Input: part model. Units: mm. Frame: model coordinates. Face numbers are marked on the shaded views. Give positions to 0.01 mm unless a question says otherwise; leave off trailing zeros. Write each loop counter-clockwise with the first axis right and the second up, starting at its lowest first coordinate (ties: lowest second). Pieces come first, ordered by that corner, then holes. Notation, with made-up numbers: (4.25, -30.5) - (41.25, -30.5) arc R15 ccw to (41.25, -11.5) - close; hole circle Ø2 at (30.25, 75). An arc over 180 degrees is marked (long way). Use a Markdown table: item, result. Add a question column.
1. Mould query, pull axis X, two halves, no side actions, for the marked faces 1 and 2. Classes: released by +X, released by -X, zero draft, split by the parting line, or undercut.
2. Pin query (flat end, axial travel): pin 1 (2 mm diameter, centred on x = 7.5, z = -20, fed in from +Y); pin 2 (0.5 mm diameter, centred on y = 1, z = -43, fed in from +X); pin 3 (1.7 mm diameter, centred on x = 1, y = 1, fed in from -Z). Return the tip coordinate at first contact, or that it passes through.
3. Section query C-C, the plane y = 3.75. Return loops of the section in (x, z), plus the area to 3 significant figures.
4. Material intervals for probe 1 along X at (y, z) = (2, -20.5); probe 2 along X at (y, z) = (0.7, 0) (1 decimal); probe 3 along Y at (x, z) = (-17, -18), sorted ascending.
5. Section query A-A, the plane z = 0. Count the separate pieces of the cut face and the enclosed holes in it, plus the area to 3 significant figures.
6. Section query B-B, the plane x = 0. Return loops of the section in (y, z) (1 decimal), plus the area to 3 significant figures.
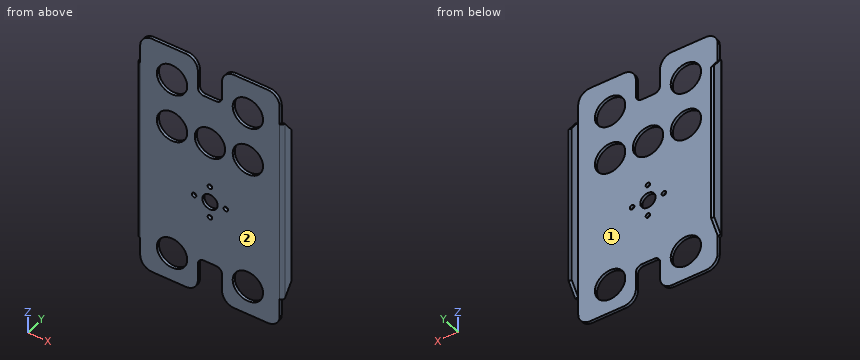
```python
from build123d import *

# Parameters (mm, degrees)
SKETCH1_R               = 7.9375
SKETCH1_R_2             = 4.0005
SKETCH1_R_3             = 1.1938
EXTRUDE1_DEPTH          = 1.524
EXTRUDE2_DEPTH          = 6.35
CUT_EXTRUDE1_DEPTH      = 39.1
CUT_EXTRUDE1_DEPTH_BACK = 39.1
FILLET1_R               = 1.5875


with BuildPart() as part:
    # Sketch1 → Extrude1 (new body)
    with BuildSketch(Plane(origin=(0, 0, 0), x_dir=(1, 0, 0), z_dir=(0, 1, 0))):
        with BuildLine():
            Line((36.4998, -62.3062), (36.4998, 36.1188))
            Line((36.4998, 36.1188), (36.4998, 39.2938))
            Line((36.4998, 39.2938), (36.4998, 45.6438))
            ThreePointArc((36.4998, 45.6438), (34.639928061, 50.133928061), (30.1498, 51.9938))
            Line((30.1498, 51.9938), (23.7998, 51.9938))
            Line((23.7998, 51.9938), (12.7, 51.9938))
            ThreePointArc((12.7, 51.9938), (8.209871939, 50.133928061), (6.35, 45.6438))
            Line((6.35, 45.6438), (6.35, 36.5252))
            ThreePointArc((6.35, 36.5252), (5.42006403, 34.28013597), (3.175, 33.3502))
            Line((3.175, 33.3502), (-3.175, 33.3502))
            ThreePointArc((-3.175, 33.3502), (-5.42006403, 34.28013597), (-6.35, 36.5252))
            Line((-6.35, 36.5252), (-6.35, 45.6438))
            ThreePointArc((-6.35, 45.6438), (-8.209871939, 50.133928061), (-12.7, 51.9938))
            Line((-12.7, 51.9938), (-23.7998, 51.9938))
            Line((-23.7998, 51.9938), (-30.1498, 51.9938))
            ThreePointArc((-30.1498, 51.9938), (-34.639928061, 50.133928061), (-36.4998, 45.6438))
            Line((-36.4998, 45.6438), (-36.4998, 39.2938))
            Line((-36.4998, 39.2938), (-36.4998, 36.1188))
            Line((-36.4998, 36.1188), (-36.4998, -62.3062))
            Line((-36.4998, -62.3062), (-36.4998, -68.6562))
            ThreePointArc((-36.4998, -68.6562), (-34.639928061, -73.146328061), (-30.1498, -75.0062))
            Line((-30.1498, -75.0062), (-23.7998, -75.0062))
            Line((-23.7998, -75.0062), (-12.7, -75.0062))
            ThreePointArc((-12.7, -75.0062), (-8.209871939, -73.146328061), (-6.35, -68.6562))
            Line((-6.35, -68.6562), (-6.35, -59.5376))
            ThreePointArc((-6.35, -59.5376), (-5.42006403, -57.29253597), (-3.175, -56.3626))
            Line((-3.175, -56.3626), (3.175, -56.3626))
            ThreePointArc((3.175, -56.3626), (5.42006403, -57.29253597), (6.35, -59.5376))
            Line((6.35, -59.5376), (6.35, -68.6562))
            ThreePointArc((6.35, -68.6562), (8.209871939, -73.146328061), (12.7, -75.0062))
            Line((12.7, -75.0062), (23.7998, -75.0062))
            Line((23.7998, -75.0062), (30.1498, -75.0062))
            ThreePointArc((30.1498, -75.0062), (34.639928061, -73.146328061), (36.4998, -68.6562))
            Line((36.4998, -68.6562), (36.4998, -62.3062))
        make_face()
        with Locations(Location((19.8374, -57.531, 0), (0, 0, 270))):  # turned: the seam where the file's is
            Circle(SKETCH1_R, mode=Mode.SUBTRACT)
        with Locations(Location((19.8374, -32.131, 0), (0, 0, 270))):  # turned: the seam where the file's is
            Circle(SKETCH1_R, mode=Mode.SUBTRACT)
        with Locations(Location((0, 0, 0), (0, 0, 270))):  # turned: the seam where the file's is
            Circle(SKETCH1_R_2, mode=Mode.SUBTRACT)
        with Locations(Location((8.3312, 0, 0), (0, 0, 270))):  # turned: the seam where the file's is
            Circle(SKETCH1_R_3, mode=Mode.SUBTRACT)
        with Locations(Location((0, -8.3312, 0), (0, 0, 270))):  # turned: the seam where the file's is
            Circle(SKETCH1_R_3, mode=Mode.SUBTRACT)
        with Locations(Location((0, 8.3312, 0), (0, 0, 270))):  # turned: the seam where the file's is
            Circle(SKETCH1_R_3, mode=Mode.SUBTRACT)
        with Locations(Location((-8.3312, 0, 0), (0, 0, 270))):  # turned: the seam where the file's is
            Circle(SKETCH1_R_3, mode=Mode.SUBTRACT)
        with Locations(Location((19.8374, 36.9062, 0), (0, 0, 270))):  # turned: the seam where the file's is
            Circle(SKETCH1_R, mode=Mode.SUBTRACT)
        with Locations(Location((0, -32.131, 0), (0, 0, 270))):  # turned: the seam where the file's is
            Circle(SKETCH1_R, mode=Mode.SUBTRACT)
        with Locations(Location((-19.8374, 36.9062, 0), (0, 0, 270))):  # turned: the seam where the file's is
            Circle(SKETCH1_R, mode=Mode.SUBTRACT)
        with Locations(Location((-19.8374, -32.131, 0), (0, 0, 270))):  # turned: the seam where the file's is
            Circle(SKETCH1_R, mode=Mode.SUBTRACT)
        with Locations(Location((-19.8374, -57.531, 0), (0, 0, 270))):  # turned: the seam where the file's is
            Circle(SKETCH1_R, mode=Mode.SUBTRACT)
    extrude(amount=EXTRUDE1_DEPTH)

    # Sketch1_3 → Extrude2 (add)
    with BuildSketch(Plane(origin=(0, 0, 0), x_dir=(1, 0, 0), z_dir=(0, 1, 0))):
        Polygon((36.4998, 36.1188), (36.4998, -59.1312), (38.1, -59.1312), (38.1, 29.7688), (38.1, 36.1188), align=None)
        Polygon((-38.1, -59.1312), (-36.4998, -59.1312), (-36.4998, 36.1188), (-38.1, 36.1188), (-38.1, 29.7688), align=None)
    extrude(amount=EXTRUDE2_DEPTH)

    # Sketch2 → Cut-Extrude1 (cut, two sides)
    with BuildSketch(Plane(origin=(0, 0, 0), x_dir=(0, 0, -1), z_dir=(1, 0, 0))) as cut_extrude1_sk:
        Polygon((-59.1312, 6.35), (-59.1312, 1.524), (-52.7812, 6.35), align=None)
        Polygon((36.1188, 6.35), (29.7688, 6.35), (36.1188, 1.524), align=None)
    extrude(amount=CUT_EXTRUDE1_DEPTH, mode=Mode.SUBTRACT)
    extrude(cut_extrude1_sk.sketch, amount=-CUT_EXTRUDE1_DEPTH_BACK, mode=Mode.SUBTRACT)

    # Fillet1
    fillet1_edges = [part.edges().sort_by_distance(p)[0] for p in [
        (38.1, 0, 11.5062),
        (-38.1, 0, 11.5062),
    ]]
    fillet(fillet1_edges, radius=FILLET1_R)


solid = part.part
```
Result sheet:
| question | item | result |
|---|---|---|
| 1 | face 1 | undercut |
| 1 | face 2 | zero draft |
| 2 | pin 1 | stops at y = 1.52 |
| 2 | pin 2 | stops at x = 36.5 |
| 2 | pin 3 | stops at z = -33.35 |
| 3 | outline | (-38.1, -33.19) - (-36.5, -33.19) - (-36.5, 56.2) - (-38.1, 56.2) - close; (36.5, -33.19) - (38.1, -33.19) - (38.1, 56.2) - (36.5, 56.2) - close |
| 3 | area | 286 mm² |
| 4 | probe 1 | x = -38.1 to -36.5, 36.5 to 38.1 |
| 4 | probe 2 | x = -37.8 to -9.5, -7.1 to -4, 4 to 7.1, 9.5 to 37.8 |
| 4 | probe 3 | y = 0 to 1.52 |
| 5 | separate pieces | 4 |
| 5 | enclosed holes | 0 |
| 5 | area | 111 mm² |
| 6 | outline | (0, -33.4) - (1.5, -33.4) - (1.5, -9.5) - (0, -9.5) - close; (0, -7.1) - (1.5, -7.1) - (1.5, -4) - (0, -4) - close; (0, 4) - (1.5, 4) - (1.5, 7.1) - (0, 7.1) - close; (0, 9.5) - (1.5, 9.5) - (1.5, 24.2) - (0, 24.2) - close; (0, 40.1) - (1.5, 40.1) - (1.5, 56.4) - (0, 56.4) - close |
| 6 | area | 93.1 mm² |
